Input: part model. Units: mm. Frame: model coordinates. A direction names the side the tool comes from. Give positions to 0.01 mm unless a question says otherwise; leave off trailing zeros. Loops run counter-clockwise (first coordinate to the right, second up) from the corner with the lowest first, then second, coordinate; pieces in that order, holes last. Notation, with made-up numbers: (-20.75, 30.25) -> (11.25, 30.25) arc R15 cw to (11.25, 42.25) -> close; hole circle Ø6 at (22.5, 58.25). An arc over 180 degrees is marked (long way). Answer in a Markdown table with one row per item. Add a question column.
```python
from build123d import *

# Parameters (mm, degrees)
SKETCH1_R           = 2.775
BOSS_EXTRUDE1_DEPTH = 44.5
SKETCH2_R           = 2.27
CUT_EXTRUDE1_DEPTH  = 5.68
CUT_EXTRUDE1_TAPER  = 3.074
SKETCH7_R           = 1
CUT_EXTRUDE2_DEPTH  = 45.5
SKETCH9_R           = 2.27
CUT_EXTRUDE3_DEPTH  = 5.68
CUT_EXTRUDE3_TAPER  = 3.074


with BuildPart() as part:
    # Sketch1 → Boss-Extrude1 (new body)
    with BuildSketch(Plane.XY):
        Circle(SKETCH1_R)
    extrude(amount=BOSS_EXTRUDE1_DEPTH)

    # Sketch2 → Cut-Extrude1 (cut)
    with BuildSketch(Plane.XY):
        Circle(SKETCH2_R)
    extrude(amount=CUT_EXTRUDE1_DEPTH, taper=CUT_EXTRUDE1_TAPER, mode=Mode.SUBTRACT)

    # Sketch7 → Cut-Extrude2 (cut, through all)
    with BuildSketch(Plane.XY):
        Circle(SKETCH7_R)
    extrude(amount=CUT_EXTRUDE2_DEPTH, mode=Mode.SUBTRACT)

    # Sketch9 → Cut-Extrude3 (cut)
    with BuildSketch(Plane.XY.offset(44.5)):
        Circle(SKETCH9_R)
    extrude(amount=-CUT_EXTRUDE3_DEPTH, taper=CUT_EXTRUDE3_TAPER, mode=Mode.SUBTRACT)


solid = part.part
```
1) Section A-A on x = 0. Output: boundary loops of the cut face in (y, z) (3 decimals).
2) Material intervals for line 1 along Y through (x, z) = (0, 23.5) (3 decimals); line 2 along Z through (x, y) = (1.7, 0.45); line 3 along X through (y, z) = (0.4, 42), sorted ascending.
3) Section C-C on z = 39.5. Output: boundary loops of the cut face in (x, y) (3 decimals), and give its area (3 significant figures).
4) Reachability of faces 1 (the face through (0, -1, 22)), 2 (the face through (1, -1, 38.82)) from +Z, -Z, +X, -X, +Y, -Y: full face, straight path, thin tool, end or side. Return the list, or none.
5) Section B-B on z = 18. Output: boundary loops of the cut face in (x, y) (3 decimals).
6) Pin query (flat end, axial travel): pin 1 (1.5 mm diameter, centred on y = 1.5, z = 35, fed in from +X); pin 2 (3 mm diameter, centred on x = 0, y = 0, fed in from -Z); pin 3 (2 mm diameter, centred on x = -1.5, z = 35, fed in from +Y). Return the tip coordinate at first contact, or that it passes through.
7) Pull-direction query (Y, two-part tool) for faces 3 (the face through (1.49, 2.34, 21.94)), 4 (the face through (1, -1, 5.68)), 5 (the face through (2.018, 0.635, 2.88)); classes: +Y half, -Y half, draft (parallel to the pull), parting line (faces both ways), or undercut.
Working result:
| question | item | result |
|---|---|---|
| 1 | outline | (-2.775, 0) -> (-2.27, 0) -> (-1.965, 5.68) -> (-1, 5.68) -> (-1, 38.82) -> (-1.965, 38.82) -> (-2.27, 44.5) -> (-2.775, 44.5) -> close; (1, 5.68) -> (1.965, 5.68) -> (2.27, 0) -> (2.775, 0) -> (2.775, 44.5) -> (2.27, 44.5) -> (1.965, 38.82) -> (1, 38.82) -> close |
| 2 | line 1 | y = -2.775 to -1, 1 to 2.775 |
| 2 | line 2 | z = 5.68 to 38.82 |
| 2 | line 3 | x = -2.75 to -2.1, 2.1 to 2.75 |
| 3 | outline | circle Ø5.55 at (0, 0); hole circle Ø4.003 at (0, 0) |
| 3 | area | 11.6 mm2 |
| 4 | face 1 | +Z, -Z |
| 4 | face 2 | +Z |
| 5 | outline | circle Ø5.55 at (0, 0); hole circle Ø2 at (0, 0) |
| 6 | pin 1 | stops at x = 2.67 |
| 6 | pin 2 | stops at z = 5.68 |
| 6 | pin 3 | stops at y = 2.73 |
| 7 | face 3 | parting line |
| 7 | face 4 | undercut |
| 7 | face 5 | undercut |
